from build123d import *

# Parameters (mm, degrees)
PAD_DEPTH     = 1.5
SKETCH001_R   = 1.7
HOLE_DEPTH    = 25
SKETCH002_R   = 2.75
HOLE001_DEPTH = 25


with BuildPart() as part:
    # Sketch → Pad (new body)
    with BuildSketch(Plane.XY):
        Polygon((-60, 11), (-60, -11), (60, -11), (60, 11), (60, 23), (48, 23), (48, 11), (-48, 11), (-48, 23), (-60, 23), align=None)
    extrude(amount=PAD_DEPTH)

    # Sketch001 (on Face8 of Pad) → Hole (cut)
    with BuildSketch(Plane.XY.offset(1.5)):
        with Locations((-45, -6)):
            Circle(SKETCH001_R)
        with Locations((-15, -6)):
            Circle(SKETCH001_R)
        with Locations((15, -6)):
            Circle(SKETCH001_R)
        with Locations((45, -6)):
            Circle(SKETCH001_R)
    extrude(amount=-HOLE_DEPTH, mode=Mode.SUBTRACT)

    # Sketch002 (on Face5 of Hole) → Hole001 (cut)
    with BuildSketch(Plane.XY.offset(1.5)):
        with Locations((52.75, 18.25)):
            Circle(SKETCH002_R)
        with Locations((-52.75, 18.25)):
            Circle(SKETCH002_R)
    extrude(amount=-HOLE001_DEPTH, mode=Mode.SUBTRACT)


solid = part.part
CAD build for the part. Positions are in the model's coordinates, mm. Coordinates: 2 decimals unless noted, no trailing zeros. Write each loop counter-clockwise with the first axis right and the second up, starting at its lowest first coordinate (ties: lowest second). Pieces come first, ordered by that corner, then holes. Notation, with made-up numbers: M 8,44 L 47,44 A9 ccw 47,56 Z; hole C -9,-26.75 d9. An arc over 180 degrees is marked long. Answer as a JSON object with one key per item and string values. Group by question number.
1) Wall check: line 1 (Y direction, x = 52.75, z = 1.15); line 2 (X direction, y = -4.5, z = 1.05); line 3 (X direction, y = 14, z = 1). Give the ranges that are in metal, low to high. Write a range as from..to.
2) Saw through at A-A (y = 13.5). Write the cut outline in (x, z), plus the area to 3 significant figures.
3) Saw through at B-B (x = -45). Write the cut outline in (y, z), plus the area to 3 significant figures.
4) Mould opens along Y. For faces 1 (the face through (16.57, -6.65, 0.76)), 2 (the face through (-1, 2, 1.5)), 3 (the face through (-46.35, -7.03, 0.76)) say: +Y half, -Y half, draft (parallel to the pull), parting line (faces both ways), or undercut.
5) Saw through at C-C (y = -6). Write the cut outline in (x, z).
6) Pin check, flat tips, straight feed: pin 1 Ø0.8 at (x, z) = (-16, 0.5) entering from +Y; pin 2 Ø5 at (x, y) = (-52.75, 18.25) entering from +Z. Stop position of each tip, or through.
7) Saw through at D-D (z = 1). Write the cut outline in (x, y).
Values follow:
{
 "1": {"line 1": "y = -11..15.5, 21..23", "line 2": "x = -60..-45.8, -44.2..-15.8, -14.2..14.2, 15.8..44.2, 45.8..60", "line 3": "x = -60..-48, 48..60"},
 "2": {"outline": "M -60,0 L -48,0 L -48,1.5 L -60,1.5 Z; M 48,0 L 60,0 L 60,1.5 L 48,1.5 Z", "area": "36.0 mm2"},
 "3": {"outline": "M -11,0 L -7.7,0 L -7.7,1.5 L -11,1.5 Z; M -4.3,0 L 11,0 L 11,1.5 L -4.3,1.5 Z", "area": "27.9 mm2"},
 "4": {"face 1": "undercut", "face 2": "draft", "face 3": "undercut"},
 "5": {"outline": "M -60,0 L -46.7,0 L -46.7,1.5 L -60,1.5 Z; M -43.3,0 L -16.7,0 L -16.7,1.5 L -43.3,1.5 Z; M -13.3,0 L 13.3,0 L 13.3,1.5 L -13.3,1.5 Z; M 16.7,0 L 43.3,0 L 43.3,1.5 L 16.7,1.5 Z; M 46.7,0 L 60,0 L 60,1.5 L 46.7,1.5 Z"},
 "6": {"pin 1": "stops at y = 11", "pin 2": "passes through"},
 "7": {"outline": "M -60,-11 L 60,-11 L 60,23 L 48,23 L 48,11 L -48,11 L -48,23 L -60,23 Z; hole C -52.75,18.25 d5.5; hole C -45,-6 d3.4; hole C -15,-6 d3.4; hole C 15,-6 d3.4; hole C 45,-6 d3.4; hole C 52.75,18.25 d5.5"}
}
